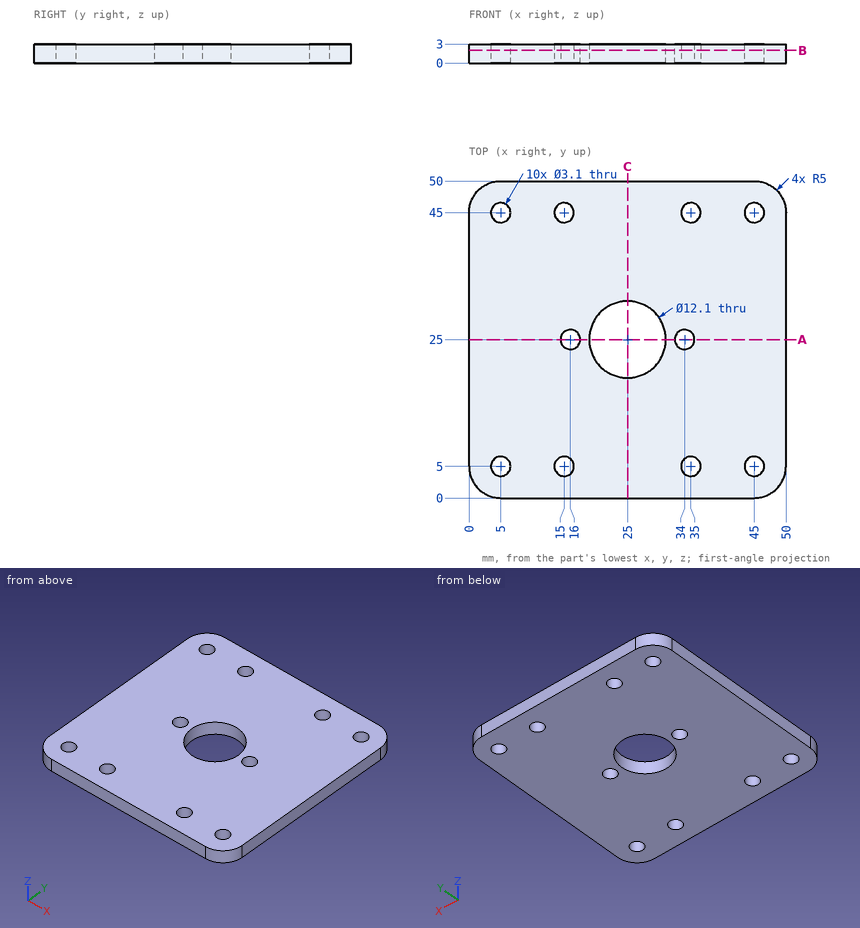
Design review of the part shown in the three views and the two pictorial views. Dimensions are in mm from the part's minimum x, y and z. Round coordinates to 2 decimals unless told otherwise and drop trailing zeros. Write each loop counter-clockwise with the first axis right and the second up, starting at its lowest first coordinate (ties: lowest second). Pieces come first, ordered by that corner, then holes.
1) For line 1 along Y through (x, z) = (5, 1.6); line 2 along Y through (x, z) = (25, 1.95); line 3 along X through (y, z) = (46, 1.5), list the stretches that pass through material, from the lowest coordinate up.
Answer below:
line 1: y = 0 to 3.45, 6.55 to 43.45, 46.55 to 50
line 2: y = 0 to 18.95, 31.05 to 50
line 3: x = 0.1 to 3.82, 6.18 to 13.82, 16.18 to 33.82, 36.18 to 43.82, 46.18 to 49.9
2) Insertion check: pin 1 Ø5 at (x, y) = (5, 5) entering from -Z. The pin has a flat end and moves straight along its axis. Give the tip position at first contact, or say it passes through.
Answer below:
pin 1: stops at z = 0
3) Take a section at C-C on x = 25. Give the boundary of the cut face in (y, z).
Answer below:
outline: (0, 0) - (18.95, 0) - (18.95, 3) - (0, 3) - close; (31.05, 0) - (50, 0) - (50, 3) - (31.05, 3) - close
4) Take a section at B-B on z = 2. State how many separate pieces and enclosed holes the cut face has, then the cut area to 3 significant figures.
Answer below:
separate pieces: 1
enclosed holes: 11
area: 2,290 mm2
5) Take a section at A-A on y = 25. Give the boundary of the cut face in (x, z), then the cut area to 3 significant figures.
Answer below:
outline: (0, 0) - (14.45, 0) - (14.45, 3) - (0, 3) - close; (17.55, 0) - (18.95, 0) - (18.95, 3) - (17.55, 3) - close; (31.05, 0) - (32.45, 0) - (32.45, 3) - (31.05, 3) - close; (35.55, 0) - (50, 0) - (50, 3) - (35.55, 3) - close
area: 95.1 mm2
